Model file for the job. Use its own axes, mm. A direction names the side the tool comes from. Round coordinates to 2 decimals unless told otherwise and drop trailing zeros. Order: outer loops, then holes, each group sorted by start corner. A loop starts at its lowest first (then second) coordinate and runs counter-clockwise, first axis right, second up. Notation, with made-up numbers: M 11,87.5 L 47,87.5 A24 cw 47,122.5 Z; hole C 76.5,-27 d9. An arc over 180 degrees is marked long. Return JSON: item names as keys, results as strings. Group by question number.
Item 1: Slice it at D-D on z = -4. Write the cut outline in (x, y), then the cut area to 3 significant figures.
Item 2: Slice it at B-B on y = -5. Write the cut outline in (x, z).
Item 3: Slice it at A-A on z = 0. Write the cut outline in (x, y), then the cut area to 3 significant figures.
Item 4: Slice it at C-C on x = 12.25. Write the cut outline in (y, z), then the cut area to 3 significant figures.
Item 5: Which spindle directions (+Z, -Z, +X, -X, +Y, -Y) get a long thin tool onto all of the face, cutting with end or side? Do faces 4 (the face through (-3.15, -6, -3)), 5 (the face through (4, -5, 5.5)), 6 (the face through (4, 0, 0)), 7 (the face through (-6, -3, 0)), 8 (the face through (2, -3, 0)). Say none if no direction does.
Item 6: Pull direction Z, two halves, no side cores. Call faces 1 (the face through (3.839, -0.285, -5.199)), 2 (the face through (4.161, -0.285, 5.199)), 3 (the face through (6, -6, -2.25)): pulls with the +Z half, pulls with the -Z half, needs draft (parallel to the pull), parting line crosses it, or undercut.
Item 7: Pin check, flat tip, straight feed: pin 1 Ø2 at (x, z) = (5, 0.5) entering from -Y. Stop position of the tip, or through.
Item 8: Probe line 1 along Z through (x, y) = (9.5, -1.1); line 2 along X through (y, z) = (-2.05, 0); line 3 along Y through (x, z) = (11.75, 0.75). List the from-to ranges inside material, lowest first.
from build123d import *

# Parameters (mm, degrees)
F0_W      = 15
F0_H      = 11
F1_DEPTH  = 10
F2_W      = 15
F2_H      = 4.5
F3_DEPTH  = 7
F4_W      = 3
F4_H      = 7
F5_DEPTH  = 7
F6_W      = 1.35
F6_H      = 8.8
F7_DEPTH  = 7.7
F9_DEPTH  = 8
F10_DEPTH = 8
F11_R     = 1
F12_R     = 1
F13_R     = 2.25
F14_DEPTH = 25


with BuildPart() as f1:
    # F0 (on Front) → F1 (new body)
    with BuildSketch(Plane.XZ):
        Rectangle(F0_W, F0_H)
    extrude(amount=F1_DEPTH)

    # F2 (on face) → F3 (cut)
    with BuildSketch(Plane.XZ.offset(10)):
        Rectangle(F2_W, F2_H)
    extrude(amount=-F3_DEPTH, mode=Mode.SUBTRACT)

    # F4 (on face) → F5 (cut)
    with BuildSketch(Plane.XZ.offset(10)):
        with Locations((-6, 0)):
            Rectangle(F4_W, F4_H)
    extrude(amount=-F5_DEPTH, mode=Mode.SUBTRACT)

    # F6 (on face) → F7 (cut)
    with BuildSketch(Plane.XZ.offset(10)):
        with Locations((-3.825, 0)):
            Rectangle(F6_W, F6_H)
    extrude(amount=-F7_DEPTH, mode=Mode.SUBTRACT)

    # F8 (on face) → F9 (join)
    with BuildSketch(Plane.YZ.offset(7.5)):
        Polygon((-10, 2.25), (-3, 2.25), (0, 2.25), (0, 5.5), (-10, 5.5), align=None)
        Polygon((0, -2.25), (-3, -2.25), (-10, -2.25), (-10, -5.5), (0, -5.5), align=None)
    extrude(amount=F9_DEPTH)

    # F10 (add): a face of the model
    f10_faces = [f1.faces().sort_by_distance(p)[0] for p in [
        (7.5, -1.5, 0),
    ]]
    extrude(f10_faces, amount=F10_DEPTH)

    # F11
    f11_edges = [f1.edges().sort_by_distance(p)[0] for p in [
        (-7.5, 0, 0),
        (4, 0, -5.5),
        (15.5, 0, 0),
        (4, 0, 5.5),
    ]]
    fillet(f11_edges, radius=F11_R)

    # F12
    f12_edges = [f1.edges().sort_by_distance(p)[0] for p in [
        (4, -10, 5.5),
        (4, -1, 5.5),
        (4, -10, -5.5),
        (4, -1, -5.5),
    ]]
    fillet(f12_edges, radius=F12_R)

    # F13 (on face) → F14 (cut)
    with BuildSketch(Plane.XZ.offset(3)):
        with Locations((9.5, 0)):
            Circle(F13_R)
    extrude(amount=-F14_DEPTH, mode=Mode.SUBTRACT)


solid = f1.part
Output values:
{
 "1": {"outline": "M -7.5,-10 L -4.5,-10 L -4.5,-2.3 L -3.15,-2.3 L -3.15,-10 L 15.5,-10 L 15.5,-1 A1 ccw 14.5,0 L -6.5,0 A1 ccw -7.5,-1 Z", "area": "219 mm²"},
 "2": {"outline": "M -7.5,-5.5 L 15.5,-5.5 L 15.5,-2.25 L -3.15,-2.25 L -3.15,-4.4 L -4.5,-4.4 L -4.5,-3.5 L -7.5,-3.5 Z; M -7.5,3.5 L -4.5,3.5 L -4.5,4.4 L -3.15,4.4 L -3.15,2.25 L 15.5,2.25 L 15.5,5.5 L -7.5,5.5 Z"},
 "3": {"outline": "M -7.5,-3 L -4.5,-3 L -4.5,-2.3 L -3.15,-2.3 L -3.15,-3 L 7.25,-3 L 7.25,0 L -6.5,0 A1 ccw -7.5,-1 Z; M 11.75,-3 L 15.5,-3 L 15.5,-1 A1 ccw 14.5,0 L 11.75,0 Z", "area": "54.1 mm²"},
 "4": {"outline": "M -10,-4.5 A1 ccw -9,-5.5 L -1,-5.5 A1 ccw 0,-4.5 L 0,4.5 A1 ccw -1,5.5 L -9,5.5 A1 ccw -10,4.5 L -10,2.25 L -3,2.25 L -3,-2.25 L -10,-2.25 Z", "area": "77.6 mm²"},
 "5": {"face 4": "-Y", "face 5": "+Z, +X, -X, +Y, -Y", "face 6": "+Z, -Z, +X, -X, +Y", "face 7": "-X, -Y", "face 8": "+X, -X, -Y"},
 "6": {"face 1": "pulls with the -Z half", "face 2": "pulls with the +Z half", "face 3": "undercut"},
 "7": {"pin 1": "y = -3"},
 "8": {"line 1": "-5.5 to -2.25, 2.25 to 5.5", "line 2": "-7.5 to 7.25, 11.75 to 15.5", "line 3": "-3 to 0"}
}
